Work out the finished part from the listing and answer in its coordinate system (mm). Face numbers are marked on the shaded views. A direction names the side the tool comes from. Coordinates: 2 decimals unless noted, no trailing zeros. Write each loop counter-clockwise with the first axis right and the second up, starting at its lowest first coordinate (ties: lowest second). Pieces come first, ordered by that corner, then holes. Notation, with made-up numbers: M -5,55.25 L 37,55.25 A20 ccw 37,72.25 Z; hole C 9.5,21.25 d5. An arc over 180 degrees is marked long. Use CSV: the item, a comma, the result in double quotes.
Autodesk Inventor part; units mm, degrees
ref_plane "YZ Plane" through (0, 0, 0) normal (1, 0, 0) x (0, 1, 0)
ref_plane "XZ Plane" through (0, 0, 0) normal (0, 1, 0) x (-1, 0, 0)
ref_plane "XY Plane" through (0, 0, 0) normal (0, 0, 1) x (1, 0, 0)
sketch "Sketch1" plane through (0, 0, 0) normal (0, 0, 1) x (1, 0, 0)
  line L0 (17.5, 25) -> (-17.5, 25)
  line L1 (-17.5, 25) -> (-17.5, -25)
  line L2 (-17.5, -25) -> (17.5, -25)
  line L3 (17.5, -25) -> (17.5, 25)
  line L4 (17.5, 25) -> (-17.5, -25) construction
  line L5 (-17.5, 25) -> (17.5, -25) construction
  line L6 (-14, -18) -> (14, -18) construction
  line L7 (14, -18) -> (14, 18) construction
  line L8 (14, 18) -> (-14, 18) construction
  line L9 (-14, 18) -> (-14, -18) construction
  line L10 (-14, -18) -> (14, 18) construction
  line L11 (14, -18) -> (-14, 18) construction
  circle A0 centre (14, 18) radius 2.4 construction
  arc A1 (13.2801, 15.7105) -> (14.7199, 15.7105) centre (14, 15.5) ccw construction
  arc A2 (14.7199, 20.2895) -> (13.2801, 20.2895) centre (14, 20.5) ccw construction
  line L12 (0, 25) -> (0, -25) construction
  line L13 (17.5, 0) -> (-17.5, 0) construction
  line L14 (0, -25) -> (0, 25) construction
  line L15 (-15, -22.5) -> (15, -22.5) construction
  line L16 (15, -22.5) -> (15, 22.5) construction
  line L17 (15, 22.5) -> (-15, 22.5) construction
  line L18 (-15, 22.5) -> (-15, -22.5) construction
  line L19 (-15, -22.5) -> (15, 22.5) construction
  line L20 (15, -22.5) -> (-15, 22.5) construction
  circle A3 centre (15, 22.5) radius 2.5 construction
  arc A4 (12.042, 23) -> (15.5, 19.542) centre (15, 22.5) ccw
  line L21 (15.5, 19.542) -> (15.5, -19.542)
  line L22 (12.042, 23) -> (-12.042, 23)
  arc A5 (-15.5, 19.542) -> (-12.042, 23) centre (-15, 22.5) ccw
  line L23 (-15.5, 19.542) -> (-15.5, -19.542)
  arc A6 (15.5, -19.542) -> (12.042, -23) centre (15, -22.5) ccw
  line L24 (12.042, -23) -> (-12.042, -23)
  arc A7 (-12.042, -23) -> (-15.5, -19.542) centre (-15, -22.5) ccw
  point P0 (0, 0)
  point P1 (14, 14.75)
  point P2 (14, 21.25)
  point P3 (13.2801, 20.2895)
  point P4 (14.7199, 20.2895)
  dimension "d0" = 35
  dimension "d1" = 50
  dimension "d2" = 4.8
  dimension "d3" = 6.5
  dimension "d4" = 1.5
  dimension "d5" = 7
  dimension "d6" = 14
  dimension "d9" = 5
  dimension "d18" = 3
  dimension "d19" = 2
  dimension "d20" = 2
extrude "Extrusion1" add sketch "Sketch1" along normal blind 1.6 contours L3 L2 L1 L0 | A4 L21 A6 L24 A7 L23 A5 L22
hole "Hole1" at (-15, -22.5, 0) at (-15, 22.5, 0) at (15, 22.5, 0) at (15, -22.5, 0) direction (0, 0, 1) diameter 2.5 end through all
fillet "Fillet1" radius 2.5 4 edges at (17.5, -25, 0.8) (-17.5, -25, 0.8) (-17.5, 25, 0.8) (17.5, 25, 0.8)
extrude "Extrusion2" add sketch "Sketch1" against normal blind 15 contours A4 L21 A6 L24 A7 L23 A5 L22
equation "\"d20\" = d19"
properties part number "SUSTAINA-USB-AUDIO-BOARD" material "CFRP"
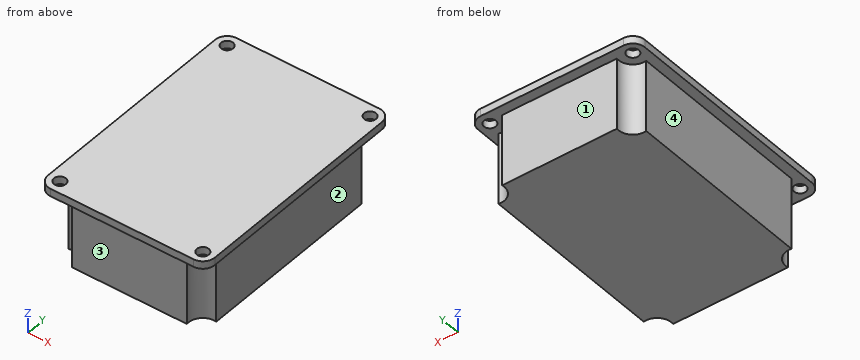
Item 1: Consider probe 1 along Y at (x, z) = (-15, 0.4); probe 2 along X at (y, z) = (22.5, 0.4); probe 3 along Y at (x, z) = (0, -2.5). Determine where each line is inside the solid, lowest interval first.
Answer:
probe 1,"y = -25 to -23.75, -21.25 to 21.25, 23.75 to 25"
probe 2,"x = -17.5 to -16.25, -13.75 to 13.75, 16.25 to 17.5"
probe 3,"y = -23 to 23"
Item 2: The part is cut by section A-A (y = -7.5). Write down the section's boundary in (x, z).
Answer:
outline,"M -17.5,0 L -15.5,0 L -15.5,-15 L 15.5,-15 L 15.5,0 L 17.5,0 L 17.5,1.6 L -17.5,1.6 Z"
Item 3: A tool of negligible diameter and unlimited length cuts with its end or side. For the marked faces 1, 2, 3 and 4, from which of +Z, -Z, +X, -X, +Y, -Y can it reach the whole face along a straight path? Write none if from no direction.
Answer:
face 1,"-Z, +X, -X, +Y"
face 2,"-Z, +X, +Y, -Y"
face 3,"-Z, +X, -X, -Y"
face 4,"-Z, -X, +Y, -Y"
Item 4: The part is cut by section B-B (x = 4). Write down the section's boundary in (y, z), then the cut area to 3 significant figures.
Answer:
outline,"M -25,0 L -23,0 L -23,-15 L 23,-15 L 23,0 L 25,0 L 25,1.6 L -25,1.6 Z"
area,"770 mm2"
Item 5: Given pin 1 (4 mm diameter, centred on y = 1, z = -4.5, fed in from -X); pin 2 (4 mm diameter, centred on x = 5, z = -6.5, fed in from -Y); pin 3 (4 mm diameter, centred on x = 15, y = 22.5, fed in from -Z); pin 4 (1.5 mm diameter, centred on x = 15, y = -22.5, fed in from +Z), each flat-ended and moving along its own axis, determine where each tip first touches the part or whether it passes through.
Answer:
pin 1,"stops at x = -15.5"
pin 2,"stops at y = -23"
pin 3,"stops at z = 0"
pin 4,"passes through"
